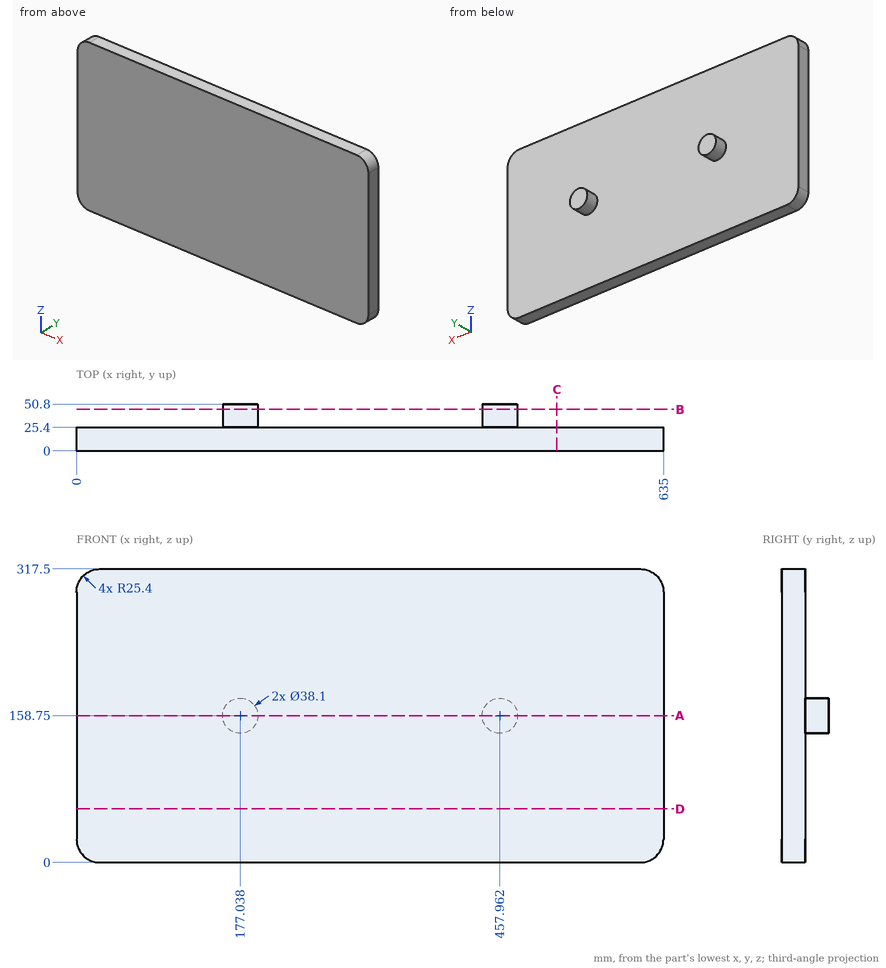
Input: dimensioned drawing with shaded views. Units: mm. Origin: part minimum x, y, z. Round coordinates to 2 decimals unless told otherwise and drop trailing zeros. Loops run counter-clockwise (first coordinate to the right, second up) from the corner with the lowest first, then second, coordinate; pieces in that order, holes last. Notation, with made-up numbers: M -39,-24 L -3,-24 A7 ccw -3,-14 Z; hole C 54,-9.5 d2. An arc over 180 degrees is marked long. Answer in a Markdown table with one row per item. Add a question column.
1. Section C-C (x = 519.5). Output: boundary loops of the cut face in (y, z), and give its area (3 significant figures).
2. Section D-D (z = 58). Output: boundary loops of the cut face in (x, y).
3. Ray query, probe 1 along Y at (x, z) = (222, 275). Return the intervals inside material, ascending.
4. Section B-B (y = 45). Output: boundary loops of the cut face in (x, z), and give its area (3 significant figures).
5. Section A-A (z = 158.75). Output: boundary loops of the cut face in (x, y), and give its area (3 significant figures).
Values follow:
| question | item | result |
|---|---|---|
| 1 | outline | M 0,0 L 25.4,0 L 25.4,317.5 L 0,317.5 Z |
| 1 | area | 8,060 mm^2 |
| 2 | outline | M 0,0 L 635,0 L 635,25.4 L 0,25.4 Z |
| 3 | probe 1 | 0 to 25.4 |
| 4 | outline | C 177.04,158.75 d38.1; C 457.96,158.75 d38.1 |
| 4 | area | 2,280 mm^2 |
| 5 | outline | M 0,0 L 635,0 L 635,25.4 L 477.01,25.4 L 477.01,50.8 L 438.91,50.8 L 438.91,25.4 L 196.09,25.4 L 196.09,50.8 L 157.99,50.8 L 157.99,25.4 L 0,25.4 Z |
| 5 | area | 18,100 mm^2 |
